Work out the finished part from the listing and answer in its coordinate system (mm). Face numbers are marked on the shaded views. Give positions to 0.01 mm unless a question says otherwise; leave off trailing zeros. Write item = value, one per line. Start each with the question number.
1. The mould has two halves that part along Y. Classify the marked faces 1, 2 and 3: released by +Y, released by -Y, zero draft, split by the parting line, or undercut.
2. A flat-ended cylindrical pin translates along its axis: pin 1 Ø0.6 at (y, z) = (0.5, 26) entering from +X. Find the tip coordinate at first contact, or state that the pin passes through.
3. Consider L1, parallel to Y at x = 20.25, z = 26; L2, parallel to Y at x = -19, z = 5.25. Determine where each line is inside the solid, lowest interval first. Write a range as [from, to].
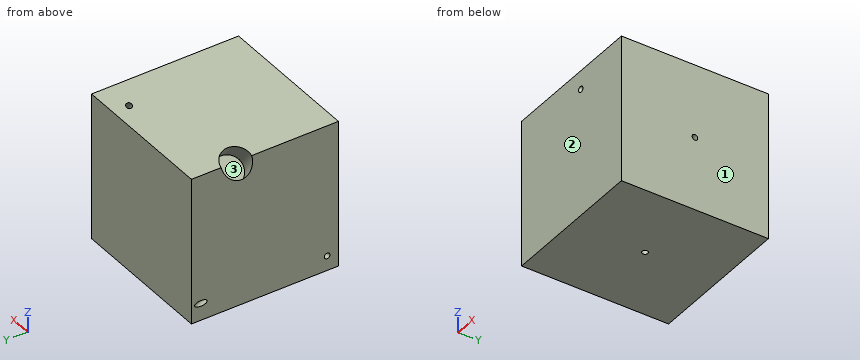
```python
from build123d import *

# Parameters (mm, degrees)
SQUARE_W             = 52
SQUARE_H             = 52
CUBE_EXTRUSION_DEPTH = 52
STICK_CUT_START      = 15
STICK_HOLE_R         = 5.1
STICK_CUT_DEPTH      = 90.048032459
SKETCH1_R            = 1
CUT_EXTRUDE1_DEPTH   = 24
SKETCH2_R            = 1
CUT_EXTRUDE2_DEPTH   = 12
SKETCH6_R            = 1
CUT_EXTRUDE4_DEPTH   = 6
SKETCH7_R            = 1
CUT_EXTRUDE5_DEPTH   = 12
SKETCH8_R            = 1
CUT_EXTRUDE6_DEPTH   = 12
SKETCH11_R           = 1
CUT_EXTRUDE7_DEPTH   = 25


with BuildPart() as part:
    # Square → Cube-Extrusion (new body)
    with BuildSketch(Plane.XY):
        Rectangle(SQUARE_W, SQUARE_H)
    extrude(amount=CUBE_EXTRUSION_DEPTH)

    # Stick-Hole → Stick-Cut (cut, through all)
    with BuildSketch(Plane(origin=(-28.888888889, 14.444444444, 28.888888889), x_dir=(-0.7453559924999299, -0.2981423969999719, -0.596284793999944), z_dir=(0.6666666666666667, -0.3333333333333332, -0.6666666666666667)).offset(STICK_CUT_START)):
        with Locations(Location((-14.635839315, -14.230249471, 0), (0, 0, 18.434948823))):
            Circle(STICK_HOLE_R)
    extrude(amount=-STICK_CUT_DEPTH, mode=Mode.SUBTRACT)

    # Sketch1 → Cut-Extrude1 (cut)
    with BuildSketch(Plane(origin=(-28.888888889, 14.444444444, 28.888888889), x_dir=(-0.7453559924999299, -0.2981423969999719, -0.596284793999944), z_dir=(0.6666666666666667, -0.3333333333333332, -0.6666666666666667))):
        with Locations(Location((-48.193677872, -5.157603573, 0), (0, 0, 36.869897646))):
            Circle(SKETCH1_R)
    extrude(amount=CUT_EXTRUDE1_DEPTH, mode=Mode.SUBTRACT)

    # Sketch2 → Cut-Extrude2 (cut)
    with BuildSketch(Plane.ZY.offset(26)):
        with Locations((5.25, -22)):
            Circle(SKETCH2_R)
    extrude(amount=-CUT_EXTRUDE2_DEPTH, mode=Mode.SUBTRACT)

    # Sketch6 → Cut-Extrude4 (cut, symmetric)
    with BuildSketch(Plane(origin=(-12.68854382, 25.37708764, 0), x_dir=(-0.894427190999916, -0.4472135954999577, 0), z_dir=(0.4472135954999577, -0.894427190999916, 0))):
        with Locations(Location((13.127553483, -6.062116333, 0), (0, 0, 180))):
            Circle(SKETCH6_R)
    extrude(amount=CUT_EXTRUDE4_DEPTH, both=True, mode=Mode.SUBTRACT)

    # Sketch7 → Cut-Extrude5 (cut)
    with BuildSketch(Plane(origin=(26, 0, 0), x_dir=(0, 0, -1), z_dir=(1, 0, 0))):
        with Locations((-26, 0)):
            Circle(SKETCH7_R)
    extrude(amount=-CUT_EXTRUDE5_DEPTH, mode=Mode.SUBTRACT)

    # Sketch8 → Cut-Extrude6 (cut)
    with BuildSketch(Plane(origin=(0, 0, 0), x_dir=(-1, 0, 0), z_dir=(0, 0, -1))):
        Circle(SKETCH8_R)
    extrude(amount=-CUT_EXTRUDE6_DEPTH, mode=Mode.SUBTRACT)

    # Sketch11 → Cut-Extrude7 (cut)
    with BuildSketch(Plane(origin=(-20.663264952, -41.326529904, 20.663264952), x_dir=(0.9128709291752769, -0.3651483716701108, 0.18257418583505525), z_dir=(0.4082482904638631, 0.8164965809277261, -0.4082482904638629))):
        with Locations(Location((22.193323836, -28.912405603, 0), (0, 0, 230.768479516))):
            Circle(SKETCH11_R)
    extrude(amount=CUT_EXTRUDE7_DEPTH, mode=Mode.SUBTRACT)


solid = part.part
```
Verdict:
q1.face_1 = zero draft
q1.face_2 = released by -Y
q1.face_3 = undercut
q2.pin_1 = 14
q3.L1 = [-26, -1], [1, 26]
q3.L2 = [-26, -23], [-21, 26]
